The listing builds one solid part. Answer for the finished solid, in the listing's coordinates (mm). A direction names the side the tool comes from. Give positions to 0.01 mm unless a question says otherwise; leave off trailing zeros. Loops run counter-clockwise (first coordinate to the right, second up) from the corner with the lowest first, then second, coordinate; pieces in that order, holes last. Notation, with made-up numbers: (-30, 18.25) - (-4, 18.25) arc R34 ccw to (-4, 56.25) - close; hole circle Ø2 at (-32.5, -17). An arc over 180 degrees is marked (long way). Answer as CSV lines item,"result". Start each with the question number.
1) Flat-ended cylindrical pins translate along their axes: pin 1 (1.5 mm diameter, centred on x = -4, z = 1.5, fed in from +Y); pin 2 (1 mm diameter, centred on x = -1.5, z = 2, fed in from +Y); pin 3 (3 mm diameter, centred on y = 0, z = 0, fed in from +X). Find the tip coordinate at first contact, or state that the pin passes through.
2) A cutting plane is placed at A-A (x = -4). Determine the outline of the cut face in (y, z) (3 decimals), and give its area (3 significant figures).
3) For faces 1 (the face through (0.35, -2.3, -1.47)), 2 (the face through (-3.531, -1.7, 3)), 3 (the face through (-3.531, -1.7, -3)), 4 (the face through (-3.531, 1.73, -2.94)), determine the directions among +Z, -Z, +X, -X, +Y, -Y from which every point of the face is accessible in a straight line to the end or side of a thin tool.
4) Find the intervals of material crossed by line 1 along Y through (x, z) = (0.1, 0); line 2 along Z through (x, y) = (-3.55, 0) (3 decimals), in increasing order.
Autodesk Inventor part; units mm, degrees
ref_plane "YZ Plane" through (0, 0, 0) normal (1, 0, 0) x (0, 1, 0)
ref_plane "XZ Plane" through (0, 0, 0) normal (0, 1, 0) x (-1, 0, 0)
ref_plane "XY Plane" through (0, 0, 0) normal (0, 0, 1) x (1, 0, 0)
sketch "Sketch1" plane through (0, 0, 0) normal (0, 0, 1) x (1, 0, 0)
  line L0 (-6.9037, 0) -> (1.1506, 0)
  line L1 (0, -3.0734) -> (0, 4.2164) construction
  line L2 (-3.5306, 3.175) -> (-5.7531, 3.175)
  line L3 (-5.7531, 3.175) -> (-5.7531, 1.2446)
  line L4 (-5.7531, 1.2446) -> (0, 1.2446)
  line L5 (0, 1.2446) -> (0, 2.7314)
  line L6 (-3.5306, 3.175) -> (-3.5306, 2.7314)
  arc A0 (0, 2.7314) -> (-3.5306, 2.7314) centre (-1.7653, -2.032) ccw
  point P0 (0, 0)
  dimension "d0" = 6.35
  dimension "d1" = 5.08
  dimension "d2" = 3.9878
  dimension "d3" = 2.2225
  dimension "d5" = 2.4892
  dimension "d6" = 5.4628
revolve "Revolution1" add sketch "Sketch1" angle 360 about axis through (-10, 0, 0) along (1, 0, 0)
sketch "Sketch2" plane through (-5.7531, 0, 0) normal (-1, 0, 0) x (0, 0, 1)
  circle A0 centre (0, 0) radius 3.175
  line L0 (3.175, -1.8331) -> (0, -3.6662)
  line L1 (0, -3.6662) -> (-3.175, -1.8331)
  line L2 (-3.175, -1.8331) -> (-3.175, 1.8331)
  line L3 (-3.175, 1.8331) -> (0, 3.6662)
  line L4 (0, 3.6662) -> (3.175, 1.8331)
  line L5 (3.175, 1.8331) -> (3.175, -1.8331)
  point P0 (3.175, 0)
extrude "Extrusion1" add sketch "Sketch2" against normal up to surface (2.2225 mm away) contours L5 L0 A0 | A0 L4 L5 | A0 L3 L4 | L0 L1 A0 | A0 L2 L3 | L1 L2 A0
sketch "Sketch3" plane through (0, 0, 0) normal (1, 0, 0) x (0, 0, -1)
  circle A0 centre (0, 0) radius 2.7314
  circle A1 centre (0, 0) radius 1.2446
extrude "Extrusion2" add sketch "Sketch3" along normal blind 0.635
fillet "Fillet1" radius 0.381 3 edges at (-3.5306, -2.7314, 0) (0, 1.9314, -1.9314) (0, -1.9314, 1.9314)
chamfer "Chamfer1" distance 0.381 angle 45 1 edges at (0.635, 0, 1.2446)
properties part number "Shock Bushing"
Ans:
1,pin 1,"y = 3.23"
1,pin 2,"y = 2.65"
1,pin 3,"x = 0.51"
2,outline,"(-3.666, 0) - (-1.833, -3.175) - (1.833, -3.175) - (3.666, 0) - (1.833, 3.175) - (-1.833, 3.175) - close; hole circle Ø2.489 at (0, 0)"
2,area,"30.1 mm2"
3,face 1,"+X"
3,face 2,"+Z, +X, -Y"
3,face 3,"-Z, +X, -Y"
3,face 4,"-Z, +X, +Y"
4,line 1,"-2.73 to -1.24, 1.24 to 2.73"
4,line 2,"-3.175 to -1.245, 1.245 to 3.175"
